Can you work these out from the model? Positions are in its coordinate system, mm. A direction names the side the tool comes from. Give positions to 0.01 mm unless a question says otherwise; leave off trailing zeros. Write each loop counter-clockwise with the first axis right and the second up, starting at its lowest first coordinate (ties: lowest second). Pieces come first, ordered by that corner, then holes. Notation, with made-up numbers: (27, 29) -> (32, 29) arc R8 ccw to (32, 42) -> close; hole circle Ø1 at (34, -30). An arc over 180 degrees is marked (long way). Answer as CSV lines item,"result". Start each with the question number.
1. I'm going to push flat-ended pins straight in: P1, Ø1.1, axis at x = 64.5, z = 0.5, coming from the +Y side; P2, Ø2.5, axis at x = 19, z = -10.5, coming from the -Y side; P3, Ø12, axis at x = 64.5, z = -5, coming from the +Y side; P4, Ø2, axis at x = 109.5, z = -11.5, coming from the -Y side. Where does each tip first touch, or does it pass through?
2. If we section it at B-B on x = 22.5: Write out the boundary of the cut face in (y, z).
3. If we section it at A-A on x = 116: Write out the boundary of the cut face in (y, z).
4. If we mould it in two halves opening along Y, with no side actions, what happens to faces 1 (the face through (10, -5.7, -12)), 2 (the face through (60, -7, 0)), 3 (the face through (64.8, -8, 0)), 4 (the face through (84, -8.7, -6))? For each: pulls with the +Y half, pulls with the -Y half, needs draft (parallel to the pull), parting line crosses it, or undercut.
5. I need wall thicknesses on line 1 (X direction, y = -13.9, z = -11.25) (3 decimals); line 2 (Z direction, x = 122, y = -8.75); line 3 (X direction, y = -8.5, z = 11.25) (3 decimals). Which ranges of each line are inside material? Lowest first, please. Write a range as [from, to].
6. On a 3-axis mill with a long thin cutter (end or side, diameter ignored), from which of +Z, -Z, +X, -X, +Y, -Y can I reach the whole of each face in a straight line? I mean faces 5 (the face through (15.438, -7.102, 2.41)), 6 (the face through (69, -5, 15)), 7 (the face through (84, -5.2, -10)), 8 (the face through (100.89, -7.5, -0.16)), 9 (the face through (70.08, -14.26, -8.4)). Say none if no direction works.
```python
from build123d import *

# Parameters (mm, degrees)
SKETCH2_W                 = 140
SKETCH2_H                 = 15
BASE_DEPTH                = 15
SKETCH3_R                 = 7.5
CENTER_CUT_DEPTH          = 142.598022585
SKETCH4_W                 = 1
SKETCH4_H                 = 25.4
ANTENNA_PCB_DEPTH         = 10.2
SKETCH14_W                = 3.5
SKETCH14_H                = 3.5
COAXIAL_CONNECTOR_DEPTH   = 3.5
LENS_START                = -23.9
SKETCH8_R                 = 9
LENS_DEPTH                = 8.6
PHOTODIODE_PCB_START      = -62.8
SKETCH10_W                = 25.4
SKETCH10_H                = 20.4
PHOTODIODE_PCB_DEPTH      = 1
FILLET1_R                 = 4.8
COAX_CONNECTOR_HOLE_START = -2
COAX_CONNECTOR_HOLE_DEPTH = 2
SKETCH16_W                = 12.7
SKETCH16_H                = 7.5
CUT_EXTRUDE2_DEPTH        = 10
BOSS_EXTRUDE1_REACH       = 143.598
CUT_EXTRUDE3_DEPTH        = 2.7
SKETCH19_R                = 1.65
CUT_EXTRUDE4_DEPTH        = 15
SKETCH20_R                = 2.85
CUT_EXTRUDE5_DEPTH        = 1.5
CUT_EXTRUDE6_REACH        = 145.962
SKETCH21_W                = 3
SKETCH21_H                = 4.5
SKETCH22_W                = 75
SKETCH22_H                = 3.5
CUT_EXTRUDE7_DEPTH        = 2
SKETCH24_W                = 3.5
SKETCH24_H                = 3.5
CUT_EXTRUDE8_DEPTH        = 15
CHAMFER2_SIZE             = 1.5
FILTER_MOUNT_START        = -56.1
FILTER_MOUNT_DEPTH        = 6.7
FILTER_SPACE_START        = -58
SKETCH9_R                 = 7
FILTER_SPACE_DEPTH        = 1.5


with BuildPart() as part:
    # Sketch2 → Base (new body)
    with BuildSketch(Plane(origin=(0, 0, 0), x_dir=(1, 0, 0), z_dir=(0, 1, 0))):
        with Locations((70, -7.5)):
            Rectangle(SKETCH2_W, SKETCH2_H)
        with Locations((70, 7.5)):
            Rectangle(SKETCH2_W, SKETCH2_H)
    extrude(amount=-BASE_DEPTH)

    # Sketch3 → Center_cut (cut, through all)
    with BuildSketch(Plane.ZY):
        Circle(SKETCH3_R)
    extrude(amount=-CENTER_CUT_DEPTH, mode=Mode.SUBTRACT)

    # Sketch4 → Antenna_PCB (cut)
    with BuildSketch(Plane(origin=(0, 0, 0), x_dir=(1, 0, 0), z_dir=(0, 1, 0))):
        with Locations((0.5, 0)):
            Rectangle(SKETCH4_W, SKETCH4_H)
    extrude(amount=-ANTENNA_PCB_DEPTH, mode=Mode.SUBTRACT)

    # Sketch14 → Coaxial_connector (cut)
    with BuildSketch(Plane.ZY.offset(-1)):
        with Locations((10.95, 0)):
            Rectangle(SKETCH14_W, SKETCH14_H)
    extrude(amount=-COAXIAL_CONNECTOR_DEPTH, mode=Mode.SUBTRACT)

    # Sketch8 → Lens (cut)
    with BuildSketch(Plane.ZY.offset(-1).offset(LENS_START)):
        Circle(SKETCH8_R)
    extrude(amount=-LENS_DEPTH, mode=Mode.SUBTRACT)

    # Sketch10 → Photodiode_PCB (cut)
    with BuildSketch(Plane.ZY.offset(-1).offset(PHOTODIODE_PCB_START)):
        Rectangle(SKETCH10_W, SKETCH10_H)
    extrude(amount=-PHOTODIODE_PCB_DEPTH, mode=Mode.SUBTRACT)

    # Fillet1
    fillet1_edges = [part.edges().sort_by_distance(p)[0] for p in [
        (70, -15, -15),
        (70, -15, 15),
    ]]
    fillet(fillet1_edges, radius=FILLET1_R)

    # Sketch15 → Coax_connector_hole (add)
    with BuildSketch(Plane(origin=(140, 0, 0), x_dir=(0, 0, -1), z_dir=(1, 0, 0)).offset(COAX_CONNECTOR_HOLE_START)):
        with BuildLine():
            ThreePointArc((-7.5, 0), (0, -7.5), (7.5, 0))
            Line((7.5, 0), (3.25, 0))
            ThreePointArc((3.25, 0), (0, -3.25), (-3.25, 0))
            Line((-3.25, 0), (-7.5, 0))
        make_face()
        with BuildLine():
            Line((11.25, -8), (11.25, 0))
            Line((11.25, 0), (7.5, 0))
            ThreePointArc((7.5, 0), (0, -7.5), (-7.5, 0))
            Line((-7.5, 0), (-11.25, 0))
            Line((-11.25, 0), (-11.25, -8))
            Line((-11.25, -8), (11.25, -8))
        make_face()
    extrude(amount=COAX_CONNECTOR_HOLE_DEPTH)

    # Sketch16 → Cut-Extrude2 (cut)
    with BuildSketch(Plane.ZY.offset(-1)):
        with Locations((-6.35, -3.75)):
            Rectangle(SKETCH16_W, SKETCH16_H)
    extrude(amount=-CUT_EXTRUDE2_DEPTH, mode=Mode.SUBTRACT)

    # Sketch17 → Boss-Extrude1 (add, up to next)
    with BuildSketch(Plane(origin=(0, 0, 0), x_dir=(1, 0, 0), z_dir=(0, 1, 0)), mode=Mode.PRIVATE) as boss_extrude1_sk1:
        Polygon((1, 12.7), (11, 8.455251838), (11, 12.7), align=None)
    boss_extrude1_tool1 = extrude(boss_extrude1_sk1.sketch, amount=-BOSS_EXTRUDE1_REACH, mode=Mode.PRIVATE) - part.part
    add(boss_extrude1_tool1.solids().sort_by_distance((7.666667, 0, -11.285084))[0])

    # Sketch18 → Cut-Extrude3 (cut)
    with BuildSketch(Plane(origin=(0, -7.5, 0), x_dir=(1, 0, 0), z_dir=(0, 1, 0))):
        Polygon((11, 8.455251838), (1, 12.7), (1, 11.830911698), (11, 7.586163536), align=None)
    extrude(amount=-CUT_EXTRUDE3_DEPTH, mode=Mode.SUBTRACT)

    # Sketch19 → Cut-Extrude4 (cut)
    with BuildSketch(Plane(origin=(0, 0, 0), x_dir=(1, 0, 0), z_dir=(0, 1, 0))):
        with Locations(Location((17.95, 11.25, 0), (0, 0, 270))):
            Circle(SKETCH19_R)
        with Locations(Location((122, 11.25, 0), (0, 0, 270))):
            Circle(SKETCH19_R)
        with Locations(Location((122, -11.25, 0), (0, 0, 39.521196359))):
            Circle(SKETCH19_R)
        with Locations(Location((17.95, -11.25, 0), (0, 0, 140.478803641))):
            Circle(SKETCH19_R)
        with Locations(Location((69.975, 11.25, 0), (0, 0, 270))):
            Circle(SKETCH19_R)
        with Locations(Location((69.975, -11.25, 0), (0, 0, 39.521196359))):
            Circle(SKETCH19_R)
    extrude(amount=-CUT_EXTRUDE4_DEPTH, mode=Mode.SUBTRACT)

    # Sketch20 → Cut-Extrude5 (cut)
    with BuildSketch(Plane.XZ.offset(15)):
        with Locations((17.95, 11.25)):
            Circle(SKETCH20_R)
        with Locations((122.05, 11.25)):
            Circle(SKETCH20_R)
        with Locations((122.05, -11.25)):
            Circle(SKETCH20_R)
        with Locations((17.95, -11.25)):
            Circle(SKETCH20_R)
        with Locations((69.975, 11.25)):
            Circle(SKETCH20_R)
        with Locations((69.975, -11.25)):
            Circle(SKETCH20_R)
    extrude(amount=-CUT_EXTRUDE5_DEPTH, mode=Mode.SUBTRACT)

    # Cut-Extrude6: up to this plane
    cut_extrude6_end = Plane(origin=(1, -15.002, -12.7), z_dir=(-0.3907311284892679, 0, 0.9205048534524428))
    # Sketch21 → Cut-Extrude6 (cut, up to the surface)
    with BuildSketch(Plane(origin=(0, 0, -15), x_dir=(-1, 0, 0), z_dir=(0, 0, -1)), mode=Mode.PRIVATE) as cut_extrude6_sk1:
        with Locations((-9.5, -7.95)):
            Rectangle(SKETCH21_W, SKETCH21_H)
    cut_extrude6_tool1 = split(extrude(cut_extrude6_sk1.sketch, amount=-CUT_EXTRUDE6_REACH, mode=Mode.PRIVATE), bisect_by=cut_extrude6_end, keep=Keep.BOTH, mode=Mode.PRIVATE)
    add(cut_extrude6_tool1.solids().sort_by_distance((9.5, -7.95, -15))[0], mode=Mode.SUBTRACT)

    # Sketch22 → Cut-Extrude7 (cut)
    with BuildSketch(Plane(origin=(0, 0, -15), x_dir=(-1, 0, 0), z_dir=(0, 0, -1))):
        with Locations((-48.5, -8.45)):
            Rectangle(SKETCH22_W, SKETCH22_H)
    extrude(amount=-CUT_EXTRUDE7_DEPTH, mode=Mode.SUBTRACT)

    # Sketch24 → Cut-Extrude8 (cut)
    with BuildSketch(Plane(origin=(0, 0, -15), x_dir=(-1, 0, 0), z_dir=(0, 0, -1))):
        with Locations((-84.25, -6.95)):
            Rectangle(SKETCH24_W, SKETCH24_H)
    extrude(amount=-CUT_EXTRUDE8_DEPTH, mode=Mode.SUBTRACT)

    # Chamfer2
    chamfer2_edges = [part.edges().sort_by_distance(p)[0] for p in [
        (84.25, -8.7, -13),
    ]]
    chamfer(chamfer2_edges, length=CHAMFER2_SIZE - 0.0001)  # a hair under: the kernel refuses the full size

    # Sketch25 → Filter_mount (add)
    with BuildSketch(Plane.ZY.offset(-1).offset(FILTER_MOUNT_START)):
        with BuildLine():
            ThreePointArc((0, -7.5), (5.303300859, -5.303300859), (7.5, 0))
            Line((7.5, 0), (5, 0))
            ThreePointArc((5, 0), (0, -5), (-5, 0))
            Line((-5, 0), (-7.5, 0))
            Line((-7.5, 0), (-7.5, -7.5))
            Line((-7.5, -7.5), (0, -7.5))
        make_face()
        with BuildLine():
            Line((7.5, -7.5), (7.5, 0))
            ThreePointArc((7.5, 0), (5.303300859, -5.303300859), (0, -7.5))
            Line((0, -7.5), (7.5, -7.5))
        make_face()
    extrude(amount=-FILTER_MOUNT_DEPTH)

    # Sketch9 → Filter_space (cut)
    with BuildSketch(Plane.ZY.offset(-1).offset(FILTER_SPACE_START)):
        Circle(SKETCH9_R)
    extrude(amount=-FILTER_SPACE_DEPTH, mode=Mode.SUBTRACT)


solid = part.part
```
Computed values:
1,P1,"stops at y = -7.44"
1,P2,"stops at y = -13.5"
1,P3,"stops at y = 0"
1,P4,"stops at y = -14.99"
2,outline,"(-15, -10.2) arc R4.8 ccw to (-10.2, -15) -> (-10.2, -13) -> (-6.7, -13) -> (-6.7, -15) -> (0, -15) -> (0, -7.5) arc R7.5 cw to (0, 7.5) -> (0, 15) -> (-10.2, 15) arc R4.8 ccw to (-15, 10.2) -> close"
3,outline,"(-15, -10.2) arc R4.8 ccw to (-10.2, -15) -> (0, -15) -> (0, -7.5) arc R7.5 cw to (0, 7.5) -> (0, 15) -> (-10.2, 15) arc R4.8 ccw to (-15, 10.2) -> close"
4,face 1,"undercut"
4,face 2,"pulls with the +Y half"
4,face 3,"needs draft"
4,face 4,"undercut"
5,line 1,"x = [0, 15.1], [20.8, 67.125], [72.825, 119.2], [124.9, 140]"
5,line 2,"z = [-15, -12.9], [-9.6, 9.6], [12.9, 15]"
5,line 3,"x = [1, 16.3], [19.6, 63.8], [64.8, 68.325], [71.625, 120.35], [123.65, 140]"
6,face 5,"-X, +Y"
6,face 6,"+Z, +X, -X, +Y, -Y"
6,face 7,"-Z"
6,face 8,"+Y"
6,face 9,"-Y"
